Verification items for this drawing (mm, ordinates from the low corner). A direction names the side the tool comes from. Coordinates: 2 decimals unless noted, no trailing zeros. Write each loop counter-clockwise with the first axis right and the second up, starting at its lowest first coordinate (ties: lowest second). Pieces come first, ordered by that corner, then holes. Notation, with made-up numbers: M -7.75,-27 L 27.25,-27 A9 cw 27.25,-17 Z; hole C -14.75,34.25 d10. An arc over 180 degrees is marked long. Put each result on its own line as item: value. Start each with the question number.
1) Cross-section at A-A on y = 17.5. Record the cut outline in (x, z).
2) Cross-section at B-B on z = 5. Record the cut outline in (x, y), plus the area to 3 significant figures.
3) Gauge pin test, flat ends, axial feed: pin 1 (4.5 mm diameter, centred on x = 10.5, y = 10.5, fed in from +Z); pin 2 (5.5 mm diameter, centred on x = 16, y = 18, fed in from +Z). Record the tip position at first contact, or that the pin passes through.
4) Set-up check for the marked faces 1, 2 and 3: record each of +Z, -Z, +X, -X, +Y, -Y from which the full face is reachable in a straight line by a thin tool's end or side.
5) Cross-section at D-D on y = 9.5. Record the cut outline in (x, z), plus the area to 3 significant figures.
6) Mould release check, pull along X, two halves, no side actions. Record for the marked faces 4, 5, 6 and 7: released by +X, released by -X, zero draft, split by the parting line, or undercut.
7) Cross-section at C-C on x = 12.5. Record the cut outline in (y, z), plus the area to 3 significant figures.
8) Scan lines: line 1 along Y through (x, z) = (12.5, 0.8); line 2 along X through (y, z) = (6.5, 3); line 3 along Z through (x, y) = (24.55, 17.5). Record each from-to range of solid material in increasing order.
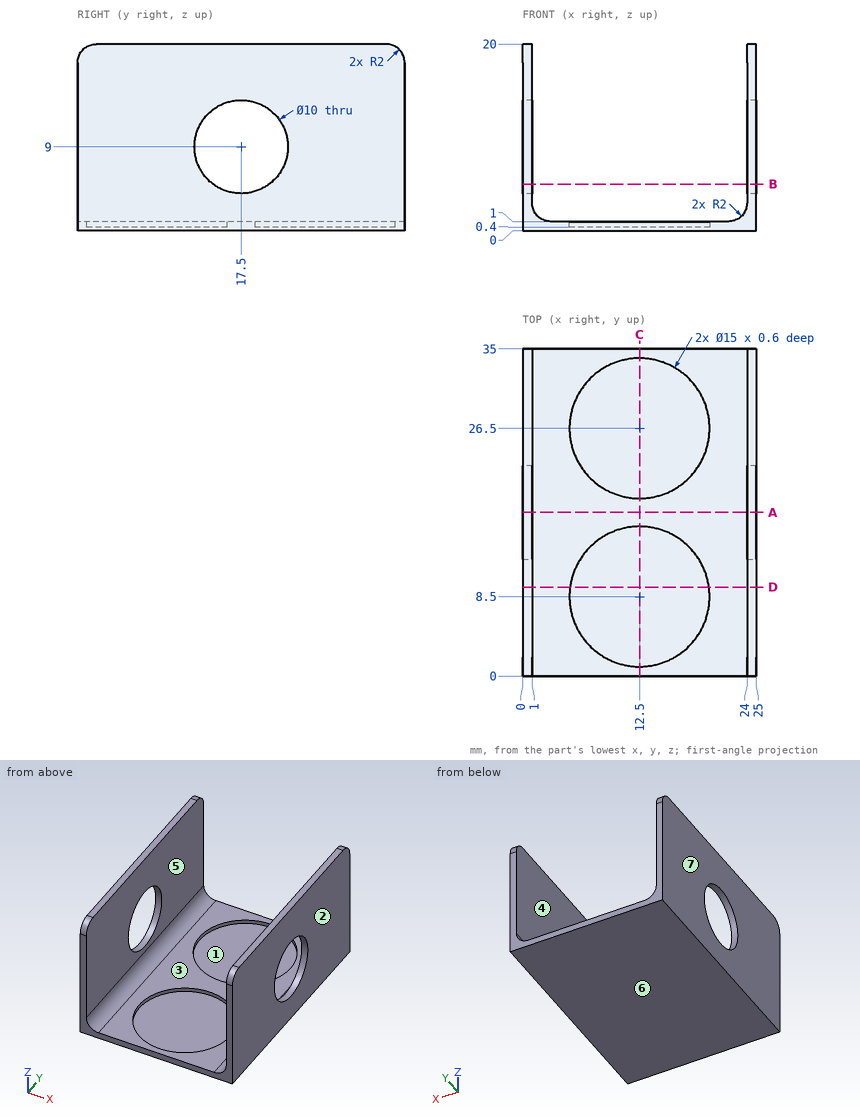
Answer key:
1. outline: M 0,0 L 25,0 L 25,4 L 24,4 L 24,3 A2 cw 22,1 L 3,1 A2 cw 1,3 L 1,4 L 0,4 Z; M 0,14 L 1,14 L 1,20 L 0,20 Z; M 24,14 L 25,14 L 25,20 L 24,20 Z
2. outline: M 0,0 L 1,0 L 1,14.5 L 0,14.5 Z; M 0,20.5 L 1,20.5 L 1,35 L 0,35 Z; M 24,0 L 25,0 L 25,14.5 L 24,14.5 Z; M 24,20.5 L 25,20.5 L 25,35 L 24,35 Z
2. area: 58.0 mm²
3. pin 1: stops at z = 0.4
3. pin 2: stops at z = 1
4. face 1: +Z
4. face 2: +Z, -Z, +X, +Y, -Y
4. face 3: +Z, +Y, -Y
5. outline: M 0,0 L 25,0 L 25,20 L 24,20 L 24,3 A2 cw 22,1 L 19.93,1 L 19.93,0.4 L 5.07,0.4 L 5.07,1 L 3,1 A2 cw 1,3 L 1,20 L 0,20 Z
5. area: 55.8 mm²
6. face 4: undercut
6. face 5: undercut
6. face 6: zero draft
6. face 7: released by -X
7. outline: M 0,0 L 35,0 L 35,1 L 34,1 L 34,0.4 L 19,0.4 L 19,1 L 16,1 L 16,0.4 L 1,0.4 L 1,1 L 0,1 Z
7. area: 17.0 mm²
8. line 1: y = 0 to 1, 16 to 19, 34 to 35
8. line 2: x = 0 to 1, 24 to 25
8. line 3: z = 0 to 4, 14 to 20
